The model under review builds one solid part; all positions refer to its coordinate system, in mm. A direction names the side the tool comes from. Give positions to 0.01 mm unless a question says otherwise; leave off trailing zeros. Loops run counter-clockwise (first coordinate to the right, second up) from the corner with the lowest first, then second, coordinate; pieces in that order, holes last. Notation, with made-up numbers: M 10,-20.5 L 37,-20.5 A23 ccw 37,-8.5 Z; hole C -38.75,76 d10. An arc over 180 degrees is marked long. Return JSON: item names as keys, results as strings.
Autodesk Inventor part; units mm, degrees
ref_plane "YZ Plane" through (0, 0, 0) normal (1, 0, 0) x (0, 1, 0)
ref_plane "XZ Plane" through (0, 0, 0) normal (0, 1, 0) x (-1, 0, 0)
ref_plane "XY Plane" through (0, 0, 0) normal (0, 0, 1) x (1, 0, 0)
sketch "Sketch1" plane through (0, 0, 0) normal (0, 1, 0) x (-1, 0, 0)
  circle A0 centre (0, 0) radius 3.5
  dimension "d0" = 7
extrude "Extrusion1" add sketch "Sketch1" along normal blind 57.5
sketch "Sketch2" plane through (0, 57.5, 0) normal (0, 1, 0) x (1, 0, 0)
  circle A0 centre (0, 0) radius 0.9252
hole "Hole1" at (0, 57.5, 0) direction (0, -1, 0) diameter 2.85 depth 19.05 tip angle 118 countersink diameter 3.048 countersink angle 82
sketch "Sketch3" plane through (0, 0, 0) normal (0, -1, 0) x (1, 0, 0)
  circle A0 centre (0, 0) radius 1.2742
hole "Hole2" at (0, 0, 0) direction (0, 1, 0) diameter 2.85 depth 19.05 tip angle 118 countersink diameter 3.048 countersink angle 82
properties part number "Connectors"
1) Consider section A-A on y = 7. Write out the cut boundary in (x, z) (3 decimals), then the cut area to 3 significant figures.
From the geometry:
{"outline": "C 0,0 d7; hole C 0,0 d2.85", "area": "32.1 mm²"}
2) Tool access review of faces 1 (the face through (0.87, 47.79, -1.13)), 2 (the face through (0.074, 19.758, -0.236)): name each direction out of +Z, -Z, +X, -X, +Y, -Y from which nothing blocks a thin tool from reaching the whole face with its end or side.
From the geometry:
{"face 1": "+Y", "face 2": "-Y"}
3) Insertion check: pin 1 (1.5 mm diameter, centred on y = 30, z = -2, fed in from -X). The pin has a flat end and moves straight along its axis. Give the tip position at first contact, or say it passes through.
From the geometry:
{"pin 1": "x = -3.27"}
4) Wall thickness on L1, parallel to Z at x = 0, y = 51.25 (3 decimals); L2, parallel to X at y = 13.5, z = -1; L3, parallel to X at y = 6, z = 0.5: over which ranges is each line inside the solid? List them lowest first. Write a range as from..to.
From the geometry:
{"L1": "-3.5..-1.425, 1.425..3.5", "L2": "-3.35..-1.02, 1.02..3.35", "L3": "-3.46..-1.33, 1.33..3.46"}
5) Consider section B-B on y = 24. Write out the cut boundary in (x, z).
From the geometry:
{"outline": "C 0,0 d7"}
6) The part is to be moulded in two halves that separate along X. For faces 3 (the face through (-1, 0, -2)), 4 (the face through (0.87, 9.71, 1.13)), 5 (the face through (-3.233, 28.348, 1.341)), say which applies: released by +X, released by -X, zero draft, split by the parting line, or undercut.
From the geometry:
{"face 3": "zero draft", "face 4": "undercut", "face 5": "split by the parting line"}
7) Consider section D-D on z = -2.25. Write out the cut boundary in (x, y).
From the geometry:
{"outline": "M -2.68,0 L 2.68,0 L 2.68,57.5 L -2.68,57.5 Z"}
8) Consider section C-C on x = -2.5. Write out the cut boundary in (y, z).
From the geometry:
{"outline": "M 0,-2.45 L 57.5,-2.45 L 57.5,2.45 L 0,2.45 Z"}
